Check sheet for the modelled part. Datum: model origin and axes. Units: mm. A direction names the side the tool comes from. Give positions to 0.01 mm unless a question says otherwise; leave off trailing zeros. Order: outer loops, then holes, each group sorted by start corner. A loop starts at its lowest first (then second) coordinate and runs counter-clockwise, first axis right, second up.
```python
from build123d import *

# Parameters (mm, degrees)
SKETCH1_W           = 30.48
SKETCH1_H           = 30.48
SKETCH1_W_2         = 25.4
SKETCH1_H_2         = 25.4
BOSS_EXTRUDE1_DEPTH = 127
BOSS_EXTRUDE2_DEPTH = 12.7


with BuildPart() as part:
    # Sketch1 → Boss-Extrude1 (new body)
    with BuildSketch(Plane.XY):
        with Locations((12.7, 12.7)):
            Rectangle(SKETCH1_W, SKETCH1_H)
        with Locations((12.7, 12.7)):
            Rectangle(SKETCH1_W_2, SKETCH1_H_2, mode=Mode.SUBTRACT)
    extrude(amount=BOSS_EXTRUDE1_DEPTH)

    # Sketch2 → Boss-Extrude2 (add, symmetric)
    with BuildSketch(Plane(origin=(12.7, 0, 0), x_dir=(0, 0, -1), z_dir=(1, 0, 0))):
        with BuildLine():
            Line((0, 27.94), (0, 33.338518846))
            Line((0, 33.338518846), (-127, 33.338518846))
            ThreePointArc((-127, 33.338518846), (-152.387152316, 57.930745818), (-128.61472889, 84.087141109))
            Line((-128.61472889, 84.087141109), (-128.61472889, 89.494679428))
            ThreePointArc((-128.61472889, 89.494679428), (-157.787927459, 57.930876659), (-127, 27.94))
            Line((-127, 27.94), (0, 27.94))
        make_face()
    extrude(amount=BOSS_EXTRUDE2_DEPTH, both=True)


solid = part.part
```
(1) Cross-section at B-B on z = 28. Enter the section's corners in (x, y).
Response values:
outline: (-2.54, -2.54) - (27.94, -2.54) - (27.94, 27.94) - (25.4, 27.94) - (25.4, 33.34) - (0, 33.34) - (0, 27.94) - (-2.54, 27.94) - close; hole (0, 0) - (25.4, 0) - (25.4, 25.4) - (0, 25.4) - close
(2) Cross-section at C-C on x = 2. Enter the section's corners in (y, z), then the cut area to 3 significant figures.
Response values:
outline: (-2.54, 0) - (0, 0) - (0, 127) - (-2.54, 127) - close; (25.4, 0) - (33.34, 0) - (33.34, 127) arc R25.4 cw to (84.09, 128.61) - (89.49, 128.61) arc R30.8 ccw to (27.94, 127) - (25.4, 127) - close
area: 1,800 mm2
(3) Cross-section at D-D on z = 144.5. Enter the section's corners in (x, y), then the cut area to 3 significant figures.
Response values:
outline: (0, 33.39) - (25.4, 33.39) - (25.4, 40.33) - (0, 40.33) - close; (0, 77.15) - (25.4, 77.15) - (25.4, 84.08) - (0, 84.08) - close
area: 352 mm2
(4) Material ranges on L1, parallel to Y at x = 9.5, z = 23.5; L2, parallel to X at y = 22.5, z = 45; L3, parallel to Z at x = 8.5, y = 60, recorded low to high.
Response values:
L1: y = -2.54 to 0, 25.4 to 33.34
L2: x = -2.54 to 0, 25.4 to 27.94
L3: z = 152.37 to 157.77
(5) Set-up check for faces 5 (the face through (13, 87, 128.615)), 6 (the face through (25.4, 32, 103)), 7 (the face through (0, 13, 63)), 8 (the face through (-1, 13, 127)): record each of +Z, -Z, +X, -X, +Y, -Y from which the full face is reachable in a straight line by a thin tool's end or side.
Response values:
face 5: -Z, +X, -X, +Y
face 6: +Z, -Z, +X, +Y
face 7: +Z, -Z
face 8: +Z, +X, -X, -Y
(6) Release check for a two-part mould opening along Y. For faces 1 (the face through (13, 25.4, 63)), 2 (the face through (12, -2.54, 63)), 3 (the face through (13, 33.339, 63)), 4 (the face through (0, 32, 103)) record: released by +Y, released by -Y, zero draft, split by the parting line, or undercut.
Response values:
face 1: undercut
face 2: released by -Y
face 3: released by +Y
face 4: zero draft
(7) Gauge pin test, flat ends, axial feed: pin 1 Ø2.5 at (x, y) = (9, 85.5) entering from -Z; pin 2 Ø12.5 at (x, z) = (17, 41.5) entering from +Y; pin 3 Ø2 at (x, y) = (10.5, 65.5) entering from +Z. Record the tip position at first contact, or that the pin passes through.
Response values:
pin 1: stops at z = 128.61
pin 2: stops at y = 33.34
pin 3: stops at z = 157.25
(8) Cross-section at A-A on y = 20. Enter the section's corners in (x, z), then the cut area to 3 significant figures.
Response values:
outline: (-2.54, 0) - (0, 0) - (0, 127) - (-2.54, 127) - close; (25.4, 0) - (27.94, 0) - (27.94, 127) - (25.4, 127) - close
area: 645 mm2
